Build history of the part. All positions in model axes, mm. A direction names the side the tool comes from. Round coordinates to 2 decimals unless told otherwise and drop trailing zeros. Write each loop counter-clockwise with the first axis right and the second up, starting at its lowest first coordinate (ties: lowest second). Pieces come first, ordered by that corner, then holes.
Item 1: Band-saw the part on A-A, the plane z = 4.5. Write the cut outline in (x, y) (3 decimals).
Item 2: Mould opens along X. For faces 5 (the cylindrical face through (-20.218, -0.181, 11.389)), 6 (the cylindrical face through (0.68, -7.05, 5.96)), 7 (the cylindrical face through (-18.373, -0.181, 9.633)) say: +X half, -X half, draft (parallel to the pull), parting line (faces both ways), or undercut.
Item 3: Drop flat-ended pins along their axis: pin 1 Ø3 at (x, y) = (-1.5, -4) entering from +Z; pin 2 Ø0.6 at (y, z) = (-0.5, 3.5) entering from +X; pin 3 Ø4 at (y, z) = (-6, 10.5) entering from +X. Give the stop position or say it passes through.
Item 4: Wall check: probe 1 along X at (y, z) = (-2.5, 6.75); probe 2 along X at (y, z) = (-2, 3.75); probe 3 along Z at (x, y) = (-15.25, -3.5). Give the ranges that are in metal, low to high.
Item 5: Band-saw the part on B-B, the plane x = -2.75. Write the cut outline in (y, z) (3 decimals), then the cut area to 3 significant figures.
Item 6: Band-saw the part on C-C, the plane y = -8.25. Write the cut outline in (x, z) (3 decimals), then the cut area to 3 significant figures.
Item 7: 3-axis set-ups, long thin cutter, end or side, ignore diameter. For faces 1 (the flat face through (0, -1, 3)), 2 (the cylindrical face through (-7.77, -9.45, 11.08)), 3 (the cylindrical face through (-7.77, -0.18, 11.08)), 4 (the flat face through (-4.902, -5, 10)): which of +Z, -Z, +X, -X, +Y, -Y reach the whole face in a straight line?
```python
from build123d import *

# Parameters (mm, degrees)
F1_DEPTH = 9.6266
F3_D     = 2.4638
F5_DEPTH = 6.1449664227
F6_R     = 0.635


# Not quite as in the source:
# - a feature names something its author has since deleted; it is built from what else it names


with BuildPart() as f1:
    # F0 (on Front) → F1 (new body)
    with BuildSketch(Plane.XZ):
        Polygon((-7.4422, 0), (0, 0), (0, 6.1449664227), (-4.9022, 6.1449664227), (-4.9022, 14.097), (-17.78, 14.097), (-22.86, 9.017), (-22.86, 0), (-20.32, 0), (-20.32, 7.4086618234), (-16.2178584248, 11.5251476239), (-8.3548940885, 11.5611667216), (-7.4422, 10.294130072), align=None)
    extrude(amount=F1_DEPTH)

    # F3 (through all)
    with Locations(Plane(origin=(0, 0, 0), x_dir=(1, 0, 0), z_dir=(0, 0, -1))):
        with Locations((-3.0988, 4.826)):
            Hole(F3_D / 2)

    # F4 (on Top) → F5 (join, through all)
    with BuildSketch(Plane.XY):
        Polygon((0, -2.032), (0, -7.5946), (2.2016586276, -6.5053654334), (2.2016586276, -3.1212345666), align=None)
    extrude(amount=F5_DEPTH)

    # F6
    f6_edges = [f1.edges().sort_by_distance(p)[0] for p in [
        (-7.4422, 0, 5.147065),
        (-7.898547, 0, 10.927648),
        (-12.286376, 0, 11.543157),
        (-20.32, 0, 3.704331),
        (-20.32, -9.6266, 3.704331),
        (-12.286376, -9.6266, 11.543157),
        (-7.898547, -9.6266, 10.927648),
        (-7.4422, -9.6266, 5.147065),
        (-4.9022, 0, 10.120983),
        (-4.9022, -9.6266, 10.120983),
        (0, -1.016, 6.144966),
        (0, -8.6106, 6.144966),
        (-2.4511, 0, 6.144966),
        (-2.4511, -9.6266, 6.144966),
        (-20.32, -9.6266, 11.557),
        (-22.86, -9.6266, 4.5085),
        (-18.268929, -9.6266, 9.466905),
        (-20.32, 0, 11.557),
        (-22.86, 0, 4.5085),
        (-18.268929, 0, 9.466905),
        (-11.3411, 0, 14.097),
        (-11.3411, -9.6266, 14.097),
        (-17.78, -4.8133, 14.097),
        (-22.86, -4.8133, 9.017),
        (1.100829, -7.049983, 6.144966),
        (2.201659, -4.8133, 6.144966),
        (1.100829, -2.576617, 6.144966),
        (2.201659, -6.505365, 3.072483),
        (2.201659, -3.121235, 3.072483),
        (-4.9022, -4.8133, 6.144966),
        (-4.9022, -4.8133, 14.097),
    ]]
    fillet(f6_edges, radius=F6_R)


solid = f1.part
```
Results:
1. outline: (-22.86, -8.992) arc R0.635 ccw to (-22.225, -9.627) - (-20.955, -9.627) arc R0.635 ccw to (-20.32, -8.992) - (-20.32, -0.635) arc R0.635 ccw to (-20.955, 0) - (-22.225, 0) arc R0.635 ccw to (-22.86, -0.635) - close; (-7.442, -8.992) arc R0.635 ccw to (-6.807, -9.627) - (0, -9.627) - (0, -7.595) - (1.848, -6.68) arc R0.635 ccw to (2.202, -6.111) - (2.202, -3.516) arc R0.635 ccw to (1.848, -2.946) - (0, -2.032) - (0, 0) - (-6.807, 0) arc R0.635 ccw to (-7.442, -0.635) - close; hole circle Ø2.464 at (-3.099, -4.826)
2. face 5: -X half
2. face 6: +X half
2. face 7: undercut
3. pin 1: stops at z = 6.14
3. pin 2: stops at x = 0
3. pin 3: stops at x = -4.9
4. probe 1: x = -22.86 to -20.32, -7.44 to -4.9
4. probe 2: x = -22.86 to -20.32, -7.44 to 0
4. probe 3: z = 11.53 to 14.1
5. outline: (-9.627, 0) - (-6.007, 0) - (-6.007, 6.145) - (-8.992, 6.145) arc R0.635 ccw to (-9.627, 5.51) - close; (-3.645, 0) - (0, 0) - (0, 5.51) arc R0.635 ccw to (-0.635, 6.145) - (-3.645, 6.145) - close
5. area: 44.5 mm2
6. outline: (-22.86, 0) - (-20.32, 0) - (-20.32, 7.409) - (-16.218, 11.525) - (-8.355, 11.561) - (-7.442, 10.294) - (-7.442, 0) - (0, 0) - (0, 5.51) arc R0.635 ccw to (-0.635, 6.145) - (-4.267, 6.145) arc R0.635 cw to (-4.902, 6.78) - (-4.902, 13.462) arc R0.635 ccw to (-5.537, 14.097) - (-17.517, 14.097) arc R0.635 ccw to (-17.966, 13.911) - (-22.674, 9.203) arc R0.635 ccw to (-22.86, 8.754) - close
6. area: 131 mm2
7. face 1: +Z, -Z, +X, +Y
7. face 2: -Z, -Y
7. face 3: -Z, +Y
7. face 4: +Z, +X, +Y, -Y
